Here's how the part is built. I have some questions about the finished solid (model axes, mm). A direction names the side the tool comes from. Round coordinates to 2 decimals unless told otherwise and drop trailing zeros. Write each loop counter-clockwise with the first axis right and the second up, starting at its lowest first coordinate (ties: lowest second). Pieces come first, ordered by that corner, then holes. Notation, with made-up numbers: (-17.5, 49.25) - (-11.5, 49.25) arc R29 cw to (-11.5, 78.25) - close; hole circle Ø2 at (80, -27.5). An arc over 180 degrees is marked (long way). Use one line per item in the form item = value. Start each with the question number.
1. If I drill on line 1 along Y through (x, z) = (0, 5.55); line 2 along Y through (x, z) = (-11.5, 5.1); line 3 along Y through (x, z) = (-19, 2.75), over which ranges is the centre line in solid material (lowest first)?
2. Which directions (+Z, -Z, +X, -X, +Y, -Y) give clear straight access to the entire face, cutting with the end or side of a thin tool? Please do faces 1 (the flat face through (11, -5, 6.5)), 2 (the flat face through (-9.96, -7.6, 10.94)), 3 (the flat face through (9.535, -7.395, 10.937)), 4 (the flat face through (0, -15, 11)), 5 (the flat face through (-10, 9, 11)).
3. We'd pull the mould along Y, two halves only. Please class faces 6 (the flat face through (-1, 9, 15.5)), 7 (the cylindrical face through (-24.5, -0.07, 4.22)), 8 (the cylindrical face through (21.5, -0.07, 4.22)), 9 (the flat face through (0, 18, 11)): +Y half, -Y half, draft (parallel to the pull), parting line (faces both ways), or undercut.
4. I want a section at B-B, the plane z = 3.75. State how many separate pieces and enclosed holes the cut face has, plus the area to 3 significant figures.
5. Will these pins go through, and if not, where does the flat tip stop? pin 1 (7.5 mm diameter, centred on x = 0, y = 3.5, fed in from +Z); pin 2 (7 mm diameter, centred on x = -3, z = 13, fed in from -Y); pin 3 (4 mm diameter, centred on x = -18.5, z = 4, fed in from -Y).
6. I want a section at A-A, the plane z = 10.25. List the corners of the cut face in (x, y) for me, plus the area to 3 significant figures.
Autodesk Inventor part; units mm, degrees
ref_plane "YZ Plane" through (0, 0, 0) normal (1, 0, 0) x (0, 1, 0)
ref_plane "XZ Plane" through (0, 0, 0) normal (0, 1, 0) x (-1, 0, 0)
ref_plane "XY Plane" through (0, 0, 0) normal (0, 0, 1) x (1, 0, 0)
sketch "Sketch1" plane through (0, 0, 0) normal (0, 0, 1) x (1, 0, 0)
  arc A0 (-8.2462, 16) -> (8.2462, 16) centre (0, 0) ccw
  line L0 (-8.2462, 16) -> (8.2462, 16)
  dimension "d0" = 36
  dimension "d1" = 16
extrude "Extrusion1" add sketch "Sketch1" along normal blind 2
sketch "Sketch2" plane through (0, 0, 2) normal (0, 0, 1) x (1, 0, 0)
  circle A0 centre (0, 0) radius 27
  circle A1 centre (0, 0) radius 23 construction
  line L0 (0, 27) -> (0, -27) construction
  line L1 (-27, 0) -> (27, 0) construction
  line L2 (8.2462, 16) -> (-8.2462, 16)
  line L3 (8.2462, 16) -> (-8.2462, 16)
  arc A2 (-8.2462, 16) -> (8.2462, 16) centre (0, 0) ccw
  circle A3 centre (0, 23) radius 1.5
  circle A4 centre (11.5, 19.9186) radius 1.5
  circle A5 centre (19.9186, 11.5) radius 1.5
  circle A6 centre (23, 0) radius 1.5
  circle A7 centre (19.9186, -11.5) radius 1.5
  circle A8 centre (11.5, -19.9186) radius 1.5
  circle A9 centre (0, -23) radius 1.5
  circle A10 centre (-11.5, -19.9186) radius 1.5
  circle A11 centre (-19.9186, -11.5) radius 1.5
  circle A12 centre (-23, 0) radius 1.5
  circle A13 centre (-19.9186, 11.5) radius 1.5
  circle A14 centre (-11.5, 19.9186) radius 1.5
  dimension "d5" = 46
  dimension "d4" = 54
  dimension "d6" = 3
  dimension "d9" = 360
extrude "Extrusion2" add sketch "Sketch2" along normal blind 4.5 contours A0 | A2 L2
chamfer "Chamfer1" distance 2 angle 45 1 edges at (0, 16, 0)
fillet "Fillet1" radius 1 2 edges at (-27, 0, 2) (-27, 0, 6.5)
sketch "Sketch3" plane through (0, 0, 0) normal (0, 0, -1) x (-1, 0, 0)
  circle A0 centre (0, 0) radius 7
  dimension "d17" = 14
hole "Hole1" at (0, 0, 0) direction (0, 0, 1) diameter 8 end through all
sketch "Sketch4" plane through (0, 0, 6.5) normal (0, 0, 1) x (1, 0, 0)
  line L0 (0, 0) -> (0, 31) construction
  line L1 (-7, 18) -> (7, 18)
  line L2 (-7, 18) -> (-13, 0)
  line L3 (0, 0) -> (0, -27) construction
  line L4 (-7, -15) -> (7, -15)
  line L5 (-7, -15) -> (-13, 0)
  line L6 (7, 18) -> (12, 0)
  line L7 (12, 0) -> (7, -15)
  line L8 (-6, 7.6667) -> (5, 7.6667)
  line L9 (5, 7.6667) -> (8, 0)
  line L10 (8, 0) -> (5.4377, -7.1718)
  line L11 (5.4377, -7.1718) -> (-5.9328, -7.1718)
  line L12 (-5.9328, -7.1718) -> (-8.7391, 0)
  line L13 (-8.7391, 0) -> (-6, 7.6667)
  point P0 (0, 18)
  dimension "d27" = 14
  dimension "d28" = 14
  dimension "d31" = 11
extrude "Extrusion4" add sketch "Sketch4" along normal blind 9
properties part number "1-26"
Model answer:
q1.line_1 = -27 to -24.5, -21.5 to -4, 4 to 21.5, 24.5 to 27
q1.line_2 = -24.43 to -21.42, -18.42 to 18.42, 21.42 to 24.43
q1.line_3 = -19.14 to -12.69, -10.31 to 10.31, 12.69 to 19.14
q2.face_1 = +Z
q2.face_2 = +Z, -X, -Y
q2.face_3 = +Z, +X, -Y
q2.face_4 = +Z, +X, -X, -Y
q2.face_5 = +Z, -X, +Y
q3.face_6 = draft
q3.face_7 = undercut
q3.face_8 = undercut
q3.face_9 = +Y half
q4.separate_pieces = 1
q4.enclosed_holes = 13
q4.area = 2,160 mm2
q5.pin_1 = 6.5
q5.pin_2 = -15
q5.pin_3 = -21.37
q6.outline = (-13, 0) - (-7, -15) - (7, -15) - (12, 0) - (7, 18) - (-7, 18) - close; hole (-8.74, 0) - (-5.93, -7.17) - (5.44, -7.17) - (8, 0) - (5, 7.67) - (-6, 7.67) - close
q6.area = 436 mm2
